The listing builds one solid part. Answer for the finished solid, in the listing's coordinates (mm). Round coordinates to 2 decimals unless told otherwise and drop trailing zeros. Write each loop counter-clockwise with the first axis right and the second up, starting at its lowest first coordinate (ties: lowest second). Pieces come first, ordered by that corner, then holes.
Item 1: Find section A-A on z = 0. Give the vertices of the cut face in (x, y), then the cut area to 3 significant figures.
Item 2: Find the intervals of material crossed by probe 1 along Z at (x, y) = (23, 2.8); probe 2 along X at (y, z) = (2.6, 0.5); probe 3 along X at (y, z) = (0.4, 3), in increasing order.
Item 3: For a pull along X with two mould halves and no side action, classify faces 1 (the face through (19.95, 1.97, 1.26)), 2 (the face through (0, 2, 15)), 3 (the face through (34.4, 2.03, 14.43)) as +X half, -X half, draft (parallel to the pull), parting line (faces both ways), or undercut.
Item 4: Find section B-B on x = 23. Give the vertices of the cut face in (y, z).
Item 5: Find section C-C on y = 1.05. Give the vertices of the cut face in (x, z).
```python
from build123d import *

# Parameters (mm, degrees)
SKETCH1_W                = 70
SKETCH1_H                = 30
BOSS_EXTRUDE1_DEPTH      = 4
FILLET1_R                = 2
M6_CLEARANCE_HOLE1_D     = 6.6
M6_CLEARANCE_HOLE1_DEPTH = 7
M6_CLEARANCE_HOLE1_TIP   = 1.982840043


with BuildPart() as part:
    # Sketch1 → Boss-Extrude1 (new body)
    with BuildSketch(Plane(origin=(0, 0, 0), x_dir=(1, 0, 0), z_dir=(0, 1, 0))):
        Rectangle(SKETCH1_W, SKETCH1_H)
    extrude(amount=BOSS_EXTRUDE1_DEPTH)

    # Fillet1
    fillet1_edges = [part.edges().sort_by_distance(p)[0] for p in [
        (-35, 2, -15),
        (35, 2, -15),
        (35, 2, 15),
        (-35, 2, 15),
    ]]
    fillet(fillet1_edges, radius=FILLET1_R)

    # M6 Clearance Hole1
    with Locations(Plane(origin=(0, 4, 0), x_dir=(1, 0, 0), z_dir=(0, 1, 0))):
        with Locations((-23, 0), (23, 0)):
            Hole(M6_CLEARANCE_HOLE1_D / 2, depth=M6_CLEARANCE_HOLE1_DEPTH)
            with Locations((0, 0, -(M6_CLEARANCE_HOLE1_DEPTH + M6_CLEARANCE_HOLE1_TIP / 2))):  # 118° drill point
                Cone(0, M6_CLEARANCE_HOLE1_D / 2, M6_CLEARANCE_HOLE1_TIP, mode=Mode.SUBTRACT)


solid = part.part
```
Check values:
1. outline: (-35, 0) - (-26.3, 0) - (-26.3, 4) - (-35, 4) - close; (-19.7, 0) - (19.7, 0) - (19.7, 4) - (-19.7, 4) - close; (26.3, 0) - (35, 0) - (35, 4) - (26.3, 4) - close
1. area: 227 mm2
2. probe 1: z = -15 to -3.3, 3.3 to 15
2. probe 2: x = -35 to -26.26, -19.74 to 19.74, 26.26 to 35
2. probe 3: x = -35 to -24.37, -21.63 to 21.63, 24.37 to 35
3. face 1: undercut
3. face 2: draft
3. face 3: +X half
4. outline: (0, -15) - (4, -15) - (4, -3.3) - (0, -3.3) - close; (0, 3.3) - (4, 3.3) - (4, 15) - (0, 15) - close
5. outline: (-35, -13) arc R2 ccw to (-33, -15) - (33, -15) arc R2 ccw to (35, -13) - (35, 13) arc R2 ccw to (33, 15) - (-33, 15) arc R2 ccw to (-35, 13) - close; hole circle Ø6.6 at (-23, 0); hole circle Ø6.6 at (23, 0)
